Could you check a few things on this drawing? It's one solid part, dimensions in mm from its lowest x, y, z. Coordinates: 2 decimals unless noted, no trailing zeros. Order: outer loops, then holes, each group sorted by start corner. A loop starts at its lowest first (then second) coordinate and runs counter-clockwise, first axis right, second up.
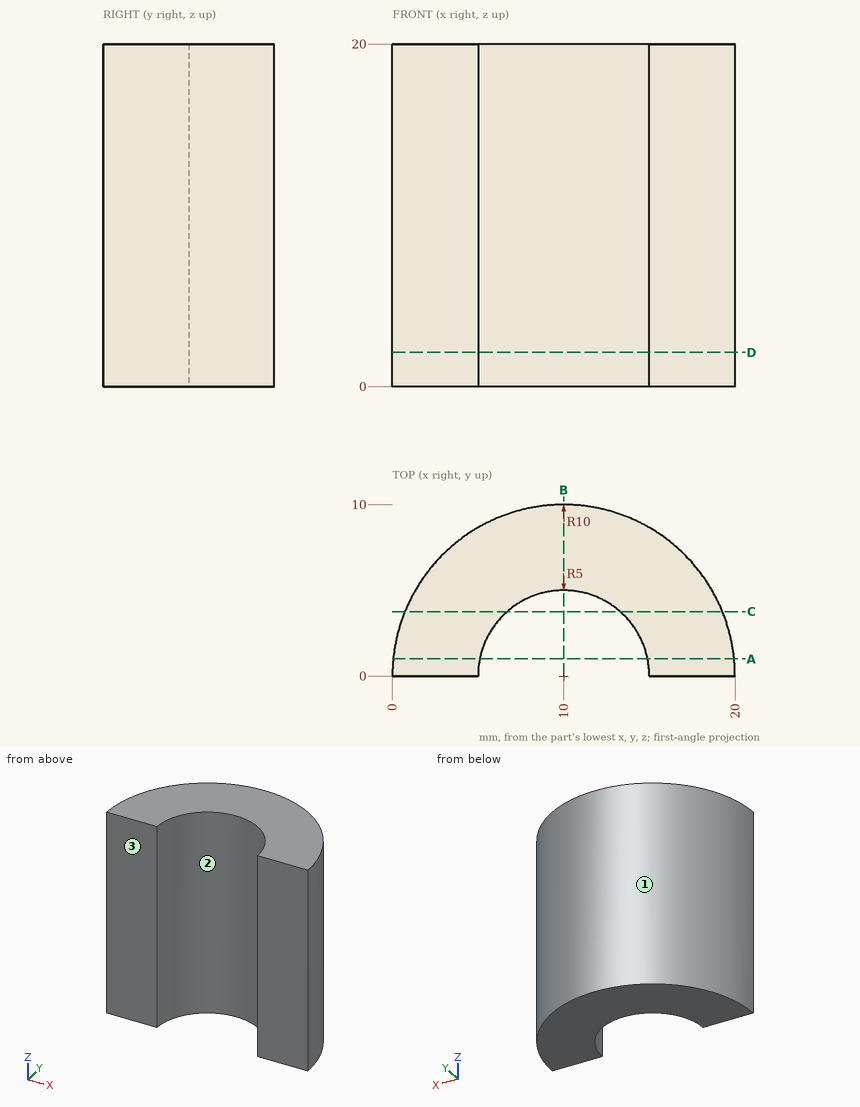
Q1. If we section it at C-C on y = 3.75: Write out the boundary of the cut face in (x, z).
Q2. Will these pins go through, and if not, where does the flat tip stop? pin 1 (1 mm diameter, centred on x = 2.5, z = 3, fed in from +Y); pin 2 (3 mm diameter, centred on x = 15.5, z = 3.5, fed in from +Y).
Q3. If we section it at A-A on y = 1: Write out the boundary of the cut face in (x, z), then the cut area to 3 significant figures.
Q4. If we section it at D-D on z = 2: Write out the boundary of the cut face in (x, y).
Q5. I need wall thicknesses on L1, parallel to X at y = 1, z = 14.5; L2, parallel to Y at x = 4.75, z = 5.75; L3, parallel to Y at x = 9.75, z = 15. Which ranges of each line are inside material? Lowest first, please.
Q6. If we section it at B-B on x = 10: Write out the boundary of the cut face in (y, z).
Q7. We'd pull the mould along X, two halves only. Please class the marked faces 1, 2 and 3: pulls with the +X half, pulls with the -X half, needs draft (parallel to the pull), parting line crosses it, or undercut.
Reply:
1. outline: (0.73, 0) - (6.69, 0) - (6.69, 20) - (0.73, 20) - close; (13.31, 0) - (19.27, 0) - (19.27, 20) - (13.31, 20) - close
2. pin 1: stops at y = 7.14
2. pin 2: stops at y = 9.17
3. outline: (0.05, 0) - (5.1, 0) - (5.1, 20) - (0.05, 20) - close; (14.9, 0) - (19.95, 0) - (19.95, 20) - (14.9, 20) - close
3. area: 202 mm2
4. outline: (0, 0) - (5, 0) arc R5 cw to (15, 0) - (20, 0) arc R10 ccw to start
5. L1: x = 0.05 to 5.1, 14.9 to 19.95
5. L2: y = 0 to 8.51
5. L3: y = 4.99 to 10
6. outline: (5, 0) - (10, 0) - (10, 20) - (5, 20) - close
7. face 1: parting line crosses it
7. face 2: undercut
7. face 3: needs draft
